Autodesk Inventor part; units mm, degrees
ref_plane "YZ Plane" through (0, 0, 0) normal (1, 0, 0) x (0, 1, 0)
ref_plane "XZ Plane" through (0, 0, 0) normal (0, 1, 0) x (-1, 0, 0)
ref_plane "XY Plane" through (0, 0, 0) normal (0, 0, 1) x (1, 0, 0)
sketch "Sketch1" plane through (0, 0, 0) normal (0, 1, 0) x (-1, 0, 0)
  circle A0 centre (0, 0) radius 10
  dimension "d0" = 20
extrude "Extrusion1" add sketch "Sketch1" along normal blind 100
sketch "Sketch2" plane through (0, 100, 0) normal (0, 1, 0) x (1, 0, 0)
  circle A0 centre (0, 0) radius 5
  dimension "d3" = 10
extrude "Extrusion2" cut sketch "Sketch2" against normal blind 30
thread "Thread1"
chamfer "Chamfer1" distance 1 angle 45 1 edges at (10, 100, 0)
chamfer "Chamfer2" distance 0.7 angle 45 1 edges at (-5, 100, 0)
sketch "Sketch8" plane through (0, 0, 0) normal (0, -1, 0) x (1, 0, 0)
  circle A0 centre (0, 0) radius 15
  dimension "d49" = 30
extrude "Extrusion3" add sketch "Sketch8" against normal blind 85
sketch "Sketch9" plane through (0, 85, 0) normal (0, 1, 0) x (1, 0, 0)
  circle A0 centre (0, 0) radius 5
extrude "Extrusion4" cut sketch "Sketch9" against normal blind 25
sketch "Sketch3" plane through (0, 70, 0) normal (0, 1, 0) x (1, 0, 0)
  point P0 (0, 0)
sketch "Sketch4" plane through (0, 70, 0) normal (0, 1, 0) x (1, 0, 0)
  point P0 (0, 0)
sketch "Sketch5" plane through (0, 70, 0) normal (0, 1, 0) x (1, 0, 0)
  point P0 (0, 0)
sketch "Sketch6" plane through (0, 70, 0) normal (0, 1, 0) x (1, 0, 0)
  point P0 (0, 0)
sketch "Sketch7" plane through (0, 70, 0) normal (0, 1, 0) x (1, 0, 0)
  point P0 (0, 0)
properties part number "rączka_korby" material "ABS Plastic"
Geometry check sheet. Reference: the model listing, model coordinates, mm. A direction names the side the tool comes from. Coordinates: 2 decimals unless noted, no trailing zeros. Order: outer loops, then holes, each group sorted by start corner. A loop starts at its lowest first (then second) coordinate and runs counter-clockwise, first axis right, second up. Notation, with made-up numbers: (53, 1.5) - (70, 1.5) arc R17 cw to (70, 7.5) - close; hole circle Ø6 at (-26, 38). An arc over 180 degrees is marked (long way). Answer as a JSON object with one key per item and string values. Group by question number.
Item 1: Sectioned sample at B-B, the plane x = 0. Record the cut outline in (y, z), and give its area (3 significant figures).
Item 2: Scan lines: probe 1 along Z at (x, y) = (0, 81); probe 2 along X at (y, z) = (80.5, -0.25); probe 3 along X at (y, z) = (87.5, 0). Record each from-to range of solid material in increasing order.
Item 3: Tool access check on faces 4 (the face through (0, 0, 0)), 5 (the face through (3, 85, -10)). Record the directions out of +Z, -Z, +X, -X, +Y, -Y that give a thin tool (end or side, any length) a straight path to the whole face; none if there is none.
Item 4: Sectioned sample at A-A, the plane z = 0. Record the cut outline in (x, y).
Item 5: Draft check along Z on faces 1 (the face through (0, 100, -6)), 2 (the face through (-14.985, 41.905, 0.66)), 3 (the face through (-1.08, 79.93, 4.88)). Enter one of: +Z half, -Z half, draft (parallel to the pull), parting line (faces both ways), or undercut.
Item 6: Sectioned sample at D-D, the plane y = 52. Record the cut outline in (x, z).
Item 7: Sectioned sample at C-C, the plane y = 67. Record the cut outline in (x, z), and give its area (3 significant figures).
Item 8: Depth check by flat-ended pin: pin 1 Ø5 at (y, z) = (31.5, 8.5) entering from +X; pin 2 Ø4 at (y, z) = (42.5, -9.5) entering from +X; pin 3 Ø5 at (y, z) = (65.5, 5.5) entering from -X. Enter the tip coordinate at first touch or a pass-through.
Resolved:
{
 "1": {"outline": "(0, -15) - (85, -15) - (85, -10) - (99, -10) - (100, -9) - (100, -5.7) - (99.3, -5) - (60, -5) - (60, 5) - (99.3, 5) - (100, 5.7) - (100, 9) - (99, 10) - (85, 10) - (85, 15) - (0, 15) - close", "area": "2,450 mm^2"},
 "2": {"probe 1": "-15 to -5, 5 to 15", "probe 2": "-15 to -4.99, 4.99 to 15", "probe 3": "-10 to -5, 5 to 10"},
 "3": {"face 4": "+Z, -Z, +X, -X, -Y", "face 5": "+Y"},
 "4": {"outline": "(-15, 0) - (15, 0) - (15, 85) - (10, 85) - (10, 99) - (9, 100) - (5.7, 100) - (5, 99.3) - (5, 60) - (-5, 60) - (-5, 99.3) - (-5.7, 100) - (-9, 100) - (-10, 99) - (-10, 85) - (-15, 85) - close"},
 "5": {"face 1": "draft", "face 2": "parting line", "face 3": "undercut"},
 "6": {"outline": "circle Ø30 at (0, 0)"},
 "7": {"outline": "circle Ø30 at (0, 0); hole circle Ø10 at (0, 0)", "area": "628 mm^2"},
 "8": {"pin 1": "x = 13.75", "pin 2": "x = 12.99", "pin 3": "x = -14.7"}
}
